```python
from build123d import *

# Parameters (mm, degrees)
SKETCH_1_W          = 48
SKETCH_1_H          = 100
EXTRUDE_1_DEPTH     = 70
SKETCH_2_W          = 44
SKETCH_2_H          = 96
CUT_EXTRUDE_1_DEPTH = 68
FILLET_1_R          = 5


with BuildPart() as part:
    # 草图1 → 凸台-拉伸1 (new body)
    with BuildSketch(Plane.XY):
        Rectangle(SKETCH_1_W, SKETCH_1_H)
    extrude(amount=EXTRUDE_1_DEPTH)

    # 草图2 → 切除-拉伸1 (cut)
    with BuildSketch(Plane(origin=(0, 0, 0), x_dir=(-1, 0, 0), z_dir=(0, 0, -1))):
        Rectangle(SKETCH_2_W, SKETCH_2_H)
    extrude(amount=-CUT_EXTRUDE_1_DEPTH, mode=Mode.SUBTRACT)

    # 圆角1
    fillet_1_edges = [part.edges().sort_by_distance(p)[0] for p in [
        (-22, 48, 34),
        (-22, -48, 34),
        (22, -48, 34),
        (22, 48, 34),
        (24, -50, 35),
        (-24, -50, 35),
        (-24, 50, 35),
        (24, 50, 35),
    ]]
    fillet(fillet_1_edges, radius=FILLET_1_R)


solid = part.part
```
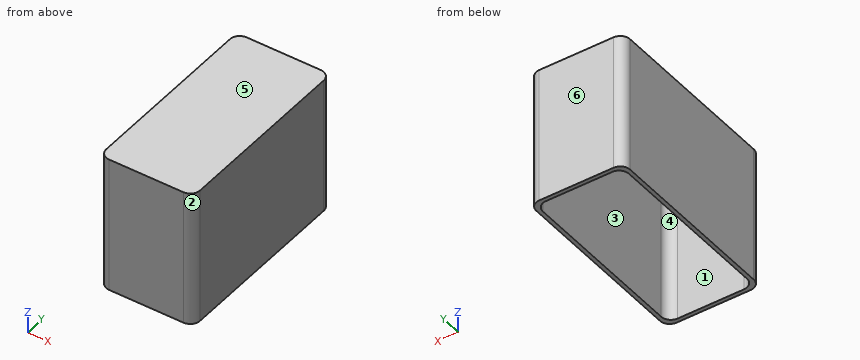
Model file for the job. Use its own axes, mm. Face numbers are marked on the shaded views. A direction names the side the tool comes from. Coordinates: 2 decimals unless noted, no trailing zeros. Write each loop counter-clockwise with the first axis right and the second up, starting at its lowest first coordinate (ties: lowest second). Pieces come first, ordered by that corner, then holes. Notation, with made-up numbers: (64.25, -5) - (119.25, -5) arc R21 ccw to (119.25, 30) - close; hole circle Ø5 at (28, -7.75). An arc over 180 degrees is marked (long way). One line per item, written item: value. Start each with the question number.
1. Slice it at B-B (x = -5.5). Write the cut outline in (y, z), plus the area to 3 significant figures.
2. Tool access for the marked faces 1 and 2: list every direction of +Z, -Z, +X, -X, +Y, -Y with a clear straight run to the whole face (end or side of a thin tool).
3. Probe line 1 (X direction, y = -12, z = 19); line 2 (Y direction, x = 16.5, z = 64.5); line 3 (Z direction, x = -8.5, y = -28.5). List the from-to ranges inside material, lowest first. Write a range as from..to.
4. Mould opens along Y. For the marked faces 3, 4, 5 and 6 say: released by +Y, released by -Y, zero draft, split by the parting line, or undercut.
5. Flat gauge pin, fed straight in: pin 1 (22 mm diameter, centred on x = 3, y = -14.5, fed in from -Z). Where does the tip first touch, or does it go through?
6. Slice it at A-A (z = 12.5). Write the cut outline in (x, y).
7. Slice it at C-C (y = 27). Write the cut outline in (x, z).
Answers below:
1. outline: (-50, 0) - (-48, 0) - (-48, 68) - (48, 68) - (48, 0) - (50, 0) - (50, 70) - (-50, 70) - close
1. area: 472 mm^2
2. face 1: -Z
2. face 2: +Z, -Z, +X, -Y
3. line 1: x = -24..-22, 22..24
3. line 2: y = -50..-48, 48..50
3. line 3: z = 68..70
4. face 3: undercut
4. face 4: undercut
4. face 5: zero draft
4. face 6: released by +Y
5. pin 1: stops at z = 68
6. outline: (-24, -45) arc R5 ccw to (-19, -50) - (19, -50) arc R5 ccw to (24, -45) - (24, 45) arc R5 ccw to (19, 50) - (-19, 50) arc R5 ccw to (-24, 45) - close; hole (-22, -43) arc R5 ccw to (-17, -48) - (17, -48) arc R5 ccw to (22, -43) - (22, 43) arc R5 ccw to (17, 48) - (-17, 48) arc R5 ccw to (-22, 43) - close
7. outline: (-24, 0) - (-22, 0) - (-22, 68) - (22, 68) - (22, 0) - (24, 0) - (24, 70) - (-24, 70) - close
